from build123d import *

# Parameters (mm, degrees)
F0_W     = 133.35
F0_H     = 25.4
F1_DEPTH = 85.09
F2_T     = -1.75
F3_DEPTH = 1.75
F4_DEPTH = 1.75


with BuildPart() as f1:
    # F0 (on Top) → F1 (new body)
    with BuildSketch(Plane.XY):
        Rectangle(F0_W, F0_H)
    extrude(amount=F1_DEPTH)

    # F2
    f2_openings = [f1.faces().sort_by_distance(p)[0] for p in [
        (0, 0, 85.09),
    ]]
    offset(amount=F2_T, openings=f2_openings)

    # F3 (cut): a face of the model
    f3_faces = [f1.faces().sort_by_distance(p)[0] for p in [
        (-66.675, 0, 42.545),
    ]]
    extrude(f3_faces, amount=-F3_DEPTH, mode=Mode.SUBTRACT)

    # F4 (cut): a face of the model
    f4_faces = [f1.faces().sort_by_distance(p)[0] for p in [
        (66.675, 0, 42.545),
    ]]
    extrude(f4_faces, amount=-F4_DEPTH, mode=Mode.SUBTRACT)


solid = f1.part
Geometry check sheet. Reference: the model listing, model coordinates, mm. A direction names the side the tool comes from. Give positions to 0.01 mm unless a question says otherwise; leave off trailing zeros. Loops run counter-clockwise (first coordinate to the right, second up) from the corner with the lowest first, then second, coordinate; pieces in that order, holes last.
(1) Depth check by flat-ended pin: pin 1 Ø4 at (x, y) = (-24.5, -1.5) entering from +Z. Enter the tip coordinate at first touch or a pass-through.
From the geometry:
pin 1: stops at z = 1.75
(2) Section check B-B on x = -54.5. Record the cut outline in (y, z).
From the geometry:
outline: (-12.7, 0) - (12.7, 0) - (12.7, 85.09) - (10.95, 85.09) - (10.95, 1.75) - (-10.95, 1.75) - (-10.95, 85.09) - (-12.7, 85.09) - close
(3) Section check C-C on y = 2.25. Record the cut outline in (x, z) (3 decimals).
From the geometry:
outline: (-64.925, 0) - (64.925, 0) - (64.925, 1.75) - (-64.925, 1.75) - close
(4) Section check A-A on z = 37. Record the cut outline in (x, y) (3 decimals).
From the geometry:
outline: (-64.925, -12.7) - (64.925, -12.7) - (64.925, -10.95) - (-64.925, -10.95) - close; (-64.925, 10.95) - (64.925, 10.95) - (64.925, 12.7) - (-64.925, 12.7) - close
(5) Thickness scan on L1, parallel to Y at x = 33.5, z = 10.5; L2, parallel to Z at x = 15, y = -4.25. Record the ranges inside material, lowest first.
From the geometry:
L1: y = -12.7 to -10.95, 10.95 to 12.7
L2: z = 0 to 1.75
(6) Set-up check for faces 1 (the flat face through (-64.925, -11.3, 36)), 2 (the flat face through (-1, 10.95, 43)): record each of +Z, -Z, +X, -X, +Y, -Y from which the full face is reachable in a straight line by a thin tool's end or side.
From the geometry:
face 1: +Z, -Z, -X, +Y, -Y
face 2: +Z, +X, -X
(7) Release check for a two-part mould opening along Y. For faces 3 (the flat face through (-1, -10.95, 43)), 4 (the flat face through (-1, -12.7, 42)), 5 (the flat face through (-1, 12.7, 42)) record: released by +Y, released by -Y, zero draft, split by the parting line, or undercut.
From the geometry:
face 3: undercut
face 4: released by -Y
face 5: released by +Y
